Input: part model. Units: mm. Frame: model coordinates. A direction names the side the tool comes from. Round coordinates to 2 decimals unless told otherwise and drop trailing zeros. Order: outer loops, then holes, each group sorted by start corner. A loop starts at its lowest first (then second) coordinate and runs counter-clockwise, first axis right, second up. Notation, with made-up numbers: (8, 29) -> (38, 29) arc R15 cw to (38, 57) -> close; hole circle Ø4 at (46, 32). An arc over 180 degrees is marked (long way). Use a Markdown table: item, result.
from build123d import *

# Parameters (mm, degrees)
SKETCH1_W           = 27.94
SKETCH1_H           = 9.144
EXTRUDE1_DEPTH      = 9.779
SKETCH2_W           = 25.654
SKETCH2_H           = 6.858
CUT_EXTRUDE1_DEPTH  = 5.588
SKETCH4_R           = 0.1905
EXTRUDE3_DEPTH      = 6.096
EXTRUDE3_DEPTH_BACK = 8


with BuildPart() as part:
    # Sketch1 → Extrude1 (new body)
    with BuildSketch(Plane.XY):
        with Locations((13.97, -4.572)):
            Rectangle(SKETCH1_W, SKETCH1_H)
    extrude(amount=EXTRUDE1_DEPTH)

    # Sketch2 → Cut-Extrude1 (cut)
    with BuildSketch(Plane.XY.offset(9.779)):
        with Locations((13.97, -4.572)):
            Rectangle(SKETCH2_W, SKETCH2_H)
    extrude(amount=-CUT_EXTRUDE1_DEPTH, mode=Mode.SUBTRACT)

    # Sketch4 → Extrude3 (add, two sides)
    with BuildSketch(Plane.XY.offset(4.191)) as extrude3_sk:
        with Locations((5.08, -5.842)):
            Circle(SKETCH4_R)
        with Locations((7.612742857, -5.842)):
            Circle(SKETCH4_R)
        with Locations((10.145485714, -5.842)):
            Circle(SKETCH4_R)
        with Locations((12.678228571, -5.842)):
            Circle(SKETCH4_R)
        with Locations((15.210971429, -5.842)):
            Circle(SKETCH4_R)
        with Locations((17.743714286, -5.842)):
            Circle(SKETCH4_R)
        with Locations((20.276457143, -5.842)):
            Circle(SKETCH4_R)
        with Locations((22.8092, -5.842)):
            Circle(SKETCH4_R)
        with Locations((5.08, -3.302)):
            Circle(SKETCH4_R)
        with Locations((7.612742857, -3.302)):
            Circle(SKETCH4_R)
        with Locations((10.145485714, -3.302)):
            Circle(SKETCH4_R)
        with Locations((12.678228571, -3.302)):
            Circle(SKETCH4_R)
        with Locations((15.210971429, -3.302)):
            Circle(SKETCH4_R)
        with Locations((17.743714286, -3.302)):
            Circle(SKETCH4_R)
        with Locations((20.276457143, -3.302)):
            Circle(SKETCH4_R)
        with Locations((22.8092, -3.302)):
            Circle(SKETCH4_R)
    extrude(amount=EXTRUDE3_DEPTH)
    extrude(extrude3_sk.sketch, amount=-EXTRUDE3_DEPTH_BACK)


solid = part.part
1) Cut plane A-A on z = 7.25. State how many separate pieces and enclosed holes the cut face has, and give its area (3 significant figures).
Answer key:
| item | result |
|---|---|
| separate pieces | 17 |
| enclosed holes | 1 |
| area | 81.4 mm^2 |
2) Cut plane B-B on x = 9. Return loops of the section in (y, z), and give its area (3 significant figures).
Answer key:
| item | result |
|---|---|
| outline | (-9.14, 0) -> (0, 0) -> (0, 9.78) -> (-1.14, 9.78) -> (-1.14, 4.19) -> (-8, 4.19) -> (-8, 9.78) -> (-9.14, 9.78) -> close |
| area | 51.1 mm^2 |
3) Ray query, probe 1 along Y at (x, z) = (22.25, 8); probe 2 along Y at (x, z) = (10, 9.5); probe 3 along Z at (x, y) = (12.5, -2.25). Return the intervals inside material, ascending.
Answer key:
| item | result |
|---|---|
| probe 1 | y = -9.14 to -8, -1.14 to 0 |
| probe 2 | y = -9.14 to -8, -5.96 to -5.72, -3.42 to -3.18, -1.14 to 0 |
| probe 3 | z = 0 to 4.19 |
4) Cut plane C-C on y = -7.5. Return loops of the section in (x, z), and give its area (3 significant figures).
Answer key:
| item | result |
|---|---|
| outline | (0, 0) -> (27.94, 0) -> (27.94, 9.78) -> (26.8, 9.78) -> (26.8, 4.19) -> (1.14, 4.19) -> (1.14, 9.78) -> (0, 9.78) -> close |
| area | 130 mm^2 |
5) Set-up query: faces 4 (the face through (14, -9.144, 5)), 5 (the face through (1.143, -5, 7)). Return all of +Z, -Z, +X, -X, +Y, -Y with unobstructed straight access to the full face (end or side cutting, diameter ignored); none if empty.
Answer key:
| item | result |
|---|---|
| face 4 | +Z, -Z, +X, -X, -Y |
| face 5 | +Z |
6) Draft query along X for faces 1 (the face through (27.94, -5, 5)), 2 (the face through (0, -5, 5)), 3 (the face through (26.797, -5, 7)). Return one class per face: released by +X, released by -X, zero draft, split by the parting line, or undercut.
Answer key:
| item | result |
|---|---|
| face 1 | released by +X |
| face 2 | released by -X |
| face 3 | undercut |
